```python
from build123d import *

# Parameters (mm, degrees)
SKETCH1_R           = 2.5
BOSS_EXTRUDE1_DEPTH = 3


with BuildPart() as part:
    # Sketch1 → Boss-Extrude1 (new body)
    with BuildSketch(Plane.XY):
        Polygon((-10, -7.5), (10, -7.5), (10, 7.5), (5.7, 7.5), (5.7, 5), (8.2, 5), (8.2, 3), (5.7, 3), (5.7, 0.5), (3.5, 0.5), (3.5, 3), (1, 3), (1, 5), (3.5, 5), (3.5, 7.5), (-3.5, 7.5), (-3.5, 5), (-1, 5), (-1, 3), (-3.5, 3), (-3.5, 0.5), (-5.7, 0.5), (-5.7, 3), (-8.2, 3), (-8.2, 5), (-5.7, 5), (-5.7, 7.5), (-10, 7.5), align=None)
        with Locations((0, -3.75)):
            Circle(SKETCH1_R, mode=Mode.SUBTRACT)
        with Locations((-6.25, -3.75)):
            Circle(SKETCH1_R, mode=Mode.SUBTRACT)
        with Locations((6.25, -3.75)):
            Circle(SKETCH1_R, mode=Mode.SUBTRACT)
    extrude(amount=BOSS_EXTRUDE1_DEPTH)


solid = part.part
```
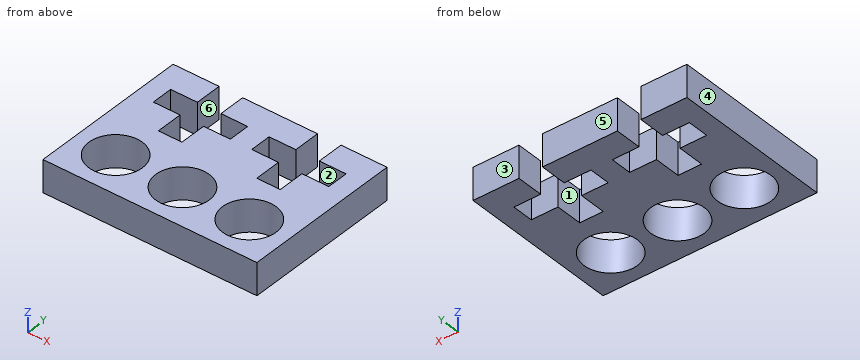
Geometry check sheet. Reference: the model listing, model coordinates, mm. Face numbers are marked on the shaded views. A direction names the side the tool comes from. Give positions to 0.01 mm unless a question says otherwise; leave off trailing zeros. Write each loop counter-clockwise with the first axis right and the second up, starting at its lowest first coordinate (ties: lowest second). Pieces come first, ordered by that corner, then holes. Notation, with made-up numbers: (22, -35.5) -> (43, -35.5) arc R20 ccw to (43, -6.5) -> close; hole circle Ø2 at (79.5, 80.5). An arc over 180 degrees is marked (long way). One line per question, with ' | ' between items.
Item 1: Draft check along X on the marked faces 4, 5 and 6. Enter one of: released by +X, released by -X, zero draft, split by the parting line, or undercut.
Determined:
face 4: released by -X | face 5: zero draft | face 6: undercut
Item 2: Access from +Z, -Z, +X, -X, +Y, -Y to the whole of each face (thin tool, end or side, straight path). Record for the marked faces 1, 2 and 3.
Determined:
face 1: +Z, -Z, +Y | face 2: +Z, -Z | face 3: +Z, -Z, +X, -X, +Y
Item 3: Sectioned sample at B-B, the plane x = 0. Record the boundary of the cut face in (y, z).
Determined:
outline: (-7.5, 0) -> (-6.25, 0) -> (-6.25, 3) -> (-7.5, 3) -> close; (-1.25, 0) -> (7.5, 0) -> (7.5, 3) -> (-1.25, 3) -> close
Item 4: Sectioned sample at D-D, the plane y = -3.75. Record the boundary of the cut face in (x, z).
Determined:
outline: (-10, 0) -> (-8.75, 0) -> (-8.75, 3) -> (-10, 3) -> close; (-3.75, 0) -> (-2.5, 0) -> (-2.5, 3) -> (-3.75, 3) -> close; (2.5, 0) -> (3.75, 0) -> (3.75, 3) -> (2.5, 3) -> close; (8.75, 0) -> (10, 0) -> (10, 3) -> (8.75, 3) -> close
Item 5: Scan lines: line 1 along Y through (x, z) = (6.25, 2.15); line 2 along X through (y, z) = (6.25, 0.25); line 3 along X through (y, z) = (4.25, 2.45). Record each from-to range of solid material in increasing order.
Determined:
line 1: -7.5 to -6.25, -1.25 to 3, 5 to 7.5 | line 2: -10 to -5.7, -3.5 to 3.5, 5.7 to 10 | line 3: -10 to -8.2, -1 to 1, 8.2 to 10
Item 6: Sectioned sample at C-C, the plane z = 0.35. State how many separate pieces and enclosed holes the cut face has, plus the area to 3 significant figures.
Determined:
separate pieces: 1 | enclosed holes: 3 | area: 190 mm^2
Item 7: Depth check by flat-ended pin: pin 1 (8 mm diameter, centred on x = 6.25, y = -3.75, fed in from +Z). Enter the tip coordinate at first touch or a pass-through.
Determined:
pin 1: z = 3
Item 8: Sectioned sample at A-A, the plane y = 5.25. Record the boundary of the cut face in (x, z), plus the area to 3 significant figures.
Determined:
outline: (-10, 0) -> (-5.7, 0) -> (-5.7, 3) -> (-10, 3) -> close; (-3.5, 0) -> (3.5, 0) -> (3.5, 3) -> (-3.5, 3) -> close; (5.7, 0) -> (10, 0) -> (10, 3) -> (5.7, 3) -> close | area: 46.8 mm^2
